Can you work these out from the drawing? Everything is in mm from the part's minimum corner. A direction names the side the tool comes from. Round coordinates to 2 decimals unless told otherwise and drop trailing zeros. Loops run counter-clockwise (first coordinate to the right, second up) from the corner with the lowest first, then second, coordinate; pieces in that order, holes last. Notation, with made-up numbers: (25.25, 31) -> (58.25, 31) arc R16 cw to (58.25, 42) -> close; hole circle Ø1 at (78, 28). An arc over 180 degrees is marked (long way). One line per item, written item: value.
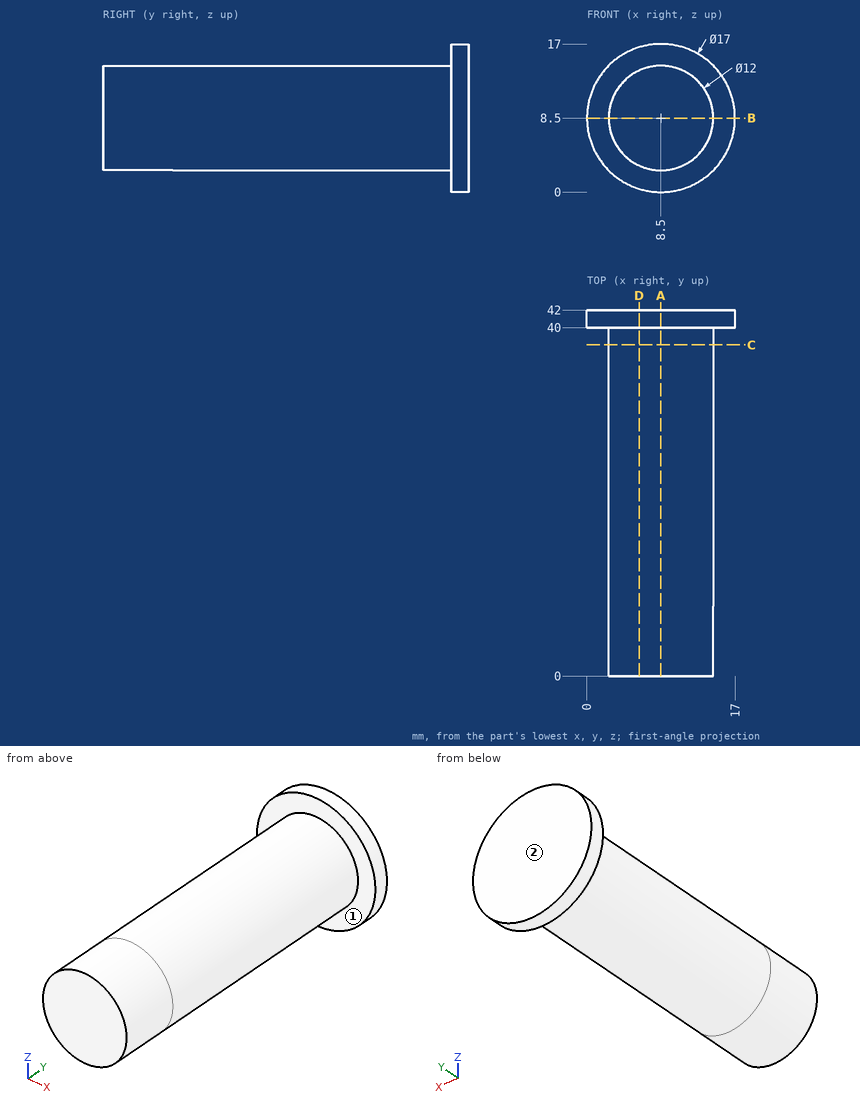
Item 1: I need wall thicknesses on line 1 (Y direction, x = 4.5, z = 3); line 2 (X direction, y = 31.5, z = 8.25); line 3 (X direction, y = 19, z = 7.5). Which ranges of each line are inside material? Lowest first, please. Write a range as from..to.
Output:
line 1: y = 40..42
line 2: x = 2.51..14.49
line 3: x = 2.58..14.42
Item 2: If we section it at B-B on z = 8.5: List the corners of the cut face in (x, y) for me.
Output:
outline: (0, 40) -> (2.5, 40) -> (2.5, 0) -> (14.5, 0) -> (14.5, 40) -> (17, 40) -> (17, 42) -> (0, 42) -> close
Item 3: For the marked faces 1 and 2, which set-ups out of +Z, -Z, +X, -X, +Y, -Y let a thin tool reach every point of the face, with its end or its side?
Output:
face 1: -Y
face 2: +Z, -Z, +X, -X, +Y
Item 4: If we section it at A-A on x = 8.5: List the corners of the cut face in (y, z) for me, plus the area to 3 significant figures.
Output:
outline: (0, 2.5) -> (40, 2.5) -> (40, 0) -> (42, 0) -> (42, 17) -> (40, 17) -> (40, 14.5) -> (0, 14.5) -> close
area: 514 mm²
Item 5: If we section it at C-C on y = 38: List the corners of the cut face in (x, z) for me, plus the area to 3 significant figures.
Output:
outline: circle Ø12 at (8.5, 8.5)
area: 113 mm²
Item 6: Will these pins go through, and if not, where does the flat tip stop? pin 1 Ø4 at (y, z) = (23.5, 6) entering from +X; pin 2 Ø2 at (y, z) = (36.5, 8) entering from -X; pin 3 Ø1 at (y, z) = (16, 13) entering from +X.
Output:
pin 1: stops at x = 14.48
pin 2: stops at x = 2.5
pin 3: stops at x = 12.97
Item 7: If we section it at D-D on x = 6: List the corners of the cut face in (y, z) for me.
Output:
outline: (0, 3.05) -> (40, 3.05) -> (40, 0.38) -> (42, 0.38) -> (42, 16.62) -> (40, 16.62) -> (40, 13.95) -> (0, 13.95) -> close
